Design review of the part built by this model. Coordinates are the model's own, in mm. Face numbers are marked on the shaded views. Round coordinates to 2 decimals unless told otherwise and drop trailing zeros. Order: outer loops, then holes, each group sorted by start corner. A loop starts at its lowest first (then second) coordinate and runs counter-clockwise, first axis right, second up. Notation, with made-up numbers: (79, -21) - (88, -21) arc R26 ccw to (88, 7) - close; hole circle Ø4 at (-24.75, -37.5). An arc over 180 degrees is marked (long way). Write item = value, one per line.
Autodesk Inventor part; units mm, degrees
ref_plane "YZ Plane" through (0, 0, 0) normal (1, 0, 0) x (0, 1, 0)
ref_plane "XZ Plane" through (0, 0, 0) normal (0, 1, 0) x (-1, 0, 0)
ref_plane "XY Plane" through (0, 0, 0) normal (0, 0, 1) x (1, 0, 0)
sketch "Sketch1" plane through (0, 0, 0) normal (1, 0, 0) x (0, 1, 0)
  circle A0 centre (0, 0) radius 86.5188
  circle A1 centre (0, 0) radius 6.35
  circle A2 centre (-38.1, 0) radius 3.175
  circle A3 centre (-19.05, -32.9956) radius 3.175
  circle A4 centre (19.05, -32.9956) radius 3.175
  circle A5 centre (38.1, 0) radius 3.175
  circle A6 centre (19.05, 32.9956) radius 3.175
  circle A7 centre (-19.05, 32.9956) radius 3.175
  circle A8 centre (-44.9072, -44.9072) radius 4.7625
  line L0 (0, 0) -> (-44.9072, -44.9072) construction
  line L1 (0, 0) -> (0, -86.5188) construction
  circle A9 centre (44.9072, -44.9072) radius 4.7625
  circle A10 centre (44.9072, 44.9072) radius 4.7625
  circle A11 centre (-44.9072, 44.9072) radius 4.7625
  dimension "d0" = 173.0375
  dimension "d1" = 12.7
  dimension "d2" = 6.35
  dimension "d3" = 38.1
  dimension "d6" = 360
  dimension "d8" = 9.525
  dimension "d9" = 45
  dimension "d13" = 360
  dimension "d26" = 89.8144
extrude "Extrusion1" add sketch "Sketch1" along normal blind 38.1
hole "Hole1" at (38.1, 0, 0) direction (-1, 0, 0) diameter 171.45 depth 37.3062
properties part number "bottom cap"
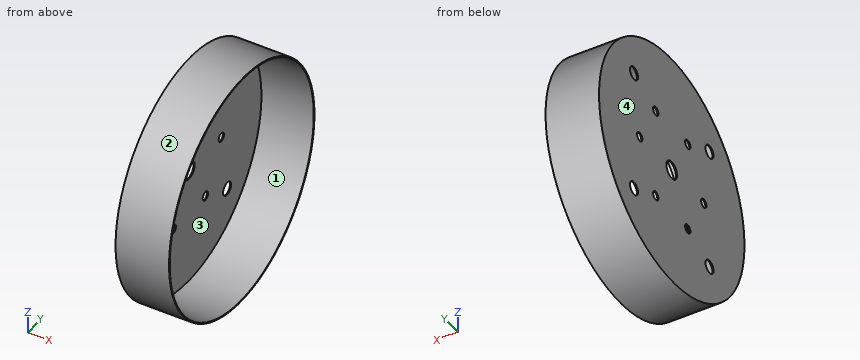
Item 1: Insertion check: P1, Ø12, axis at y = 22.5, z = -39, coming from the +X side; P2, Ø4, axis at x = 26, z = 26, coming from the +Y side; P3, Ø5.5, axis at y = -19.05, z = 33, coming from the +X side; P4, Ø6, axis at x = 24.5, y = 60, coming from the -Z side. Each pin has a flat end and moves straight along its axis. Give the tip position at first contact, or say it passes through.
Data:
P1 = 0.79
P2 = 83.12
P3 = through
P4 = -65.09
Item 2: Take a section at D-D, the plane x = 23. State the section outline as (y, z) points (3 decimals), and give its area (3 significant figures).
Data:
outline = circle Ø173.038 at (0, 0); hole circle Ø171.45 at (0, 0)
area = 430 mm2
Item 3: The part is to be moulded in two halves that separate along Z. For the marked faces 1, 2, 3 and 4, say which applies: +Z half, -Z half, draft (parallel to the pull), parting line (faces both ways), or undercut.
Data:
face_1 = undercut
face_2 = parting line
face_3 = undercut
face_4 = draft
Item 4: Take a section at B-B, the plane y = 19.05. State the section outline as (x, z) points, and give its area (3 significant figures).
Data:
outline = (0, -84.4) - (38.1, -84.4) - (38.1, -83.58) - (0.79, -83.58) - (0.79, -36.17) - (0, -36.17) - close; (0, -29.82) - (0.79, -29.82) - (0.79, 29.82) - (0, 29.82) - close; (0, 36.17) - (0.79, 36.17) - (0.79, 83.58) - (38.1, 83.58) - (38.1, 84.4) - (0, 84.4) - close
area = 185 mm2
Item 5: Take a section at A-A, the plane y = 0. State the section outline as (x, z) points (3 decimals).
Data:
outline = (0, -86.519) - (38.1, -86.519) - (38.1, -85.725) - (0.794, -85.725) - (0.794, -6.35) - (0, -6.35) - close; (0, 6.35) - (0.794, 6.35) - (0.794, 85.725) - (38.1, 85.725) - (38.1, 86.519) - (0, 86.519) - close
Item 6: For line 1 along X through (y, z) = (25.5, -7.5); line 2 along Y through (x, z) = (4.5, 52.5); line 3 along Z through (x, y) = (13, 52), list the stretches that pass through material, from the lowest coordinate up. Write a range as [from, to].
Data:
line_1 = [0, 0.79]
line_2 = [-68.77, -67.77], [67.77, 68.77]
line_3 = [-69.15, -68.15], [68.15, 69.15]
Item 7: Take a section at C-C, the plane z = 61. State the section outline as (x, y) points, and give its area (3 significant figures).
Data:
outline = (0, -61.36) - (38.1, -61.36) - (38.1, -60.23) - (0.79, -60.23) - (0.79, 60.23) - (38.1, 60.23) - (38.1, 61.36) - (0, 61.36) - close
area = 181 mm2
